The figure shows three views and two pictorial views of one solid part (mm, origin at its lowest corner). Answer the questions. A direction names the side the tool comes from. Coordinates: 2 decimals unless noted, no trailing zeros. Order: outer loops, then holes, each group sorted by start corner. A loop starts at its lowest first (then second) coordinate and runs counter-clockwise, first axis right, second up. Notation, with made-up numbers: (39.25, 1.5) - (52.25, 1.5) arc R21 ccw to (52.25, 7.5) - close; hole circle Ø6 at (-32, 17). An arc over 180 degrees is marked (long way). Answer as a JSON object with one key per item and string values. Group by question number.
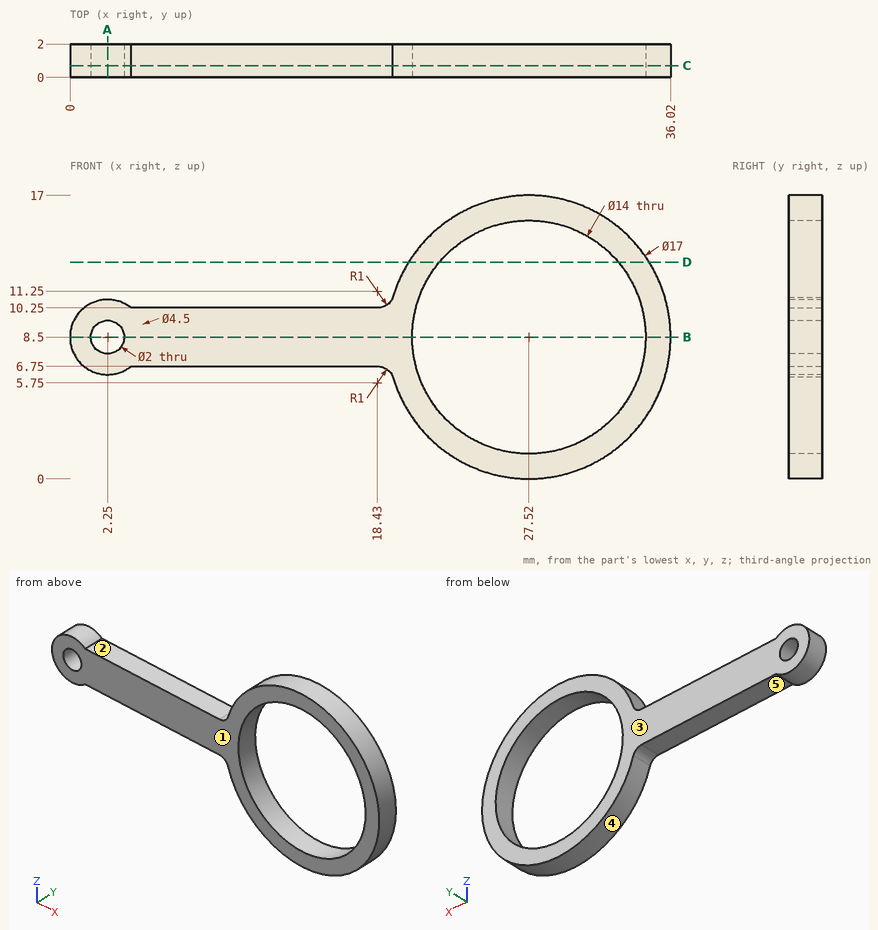
1. A cutting plane is placed at D-D on z = 13. Write down the section's boundary in (x, y), and give its area (3 significant figures).
2. Given pin 1 (1 mm diameter, centred on x = 21.5, y = 1.5, fed in from -Z); pin 2 (1 mm diameter, centred on x = 8.5, y = 1.5, fed in from +Z), each flat-ended and moving along its own axis, determine where each tip first touches the part or whether it passes through.
3. For a pull along X with two mould halves and no side action, classify the marked faces 3, 4 and 5 as pulls with the +X half, pulls with the -X half, needs draft (parallel to the pull), parting line crosses it, or undercut.
4. A cutting plane is placed at B-B on z = 8.5. Write down the section's boundary in (x, y), and give its area (3 significant figures).
5. Straight lines are drawn through the part: L1, parallel to X at y = 0.65, z = 8.5; L2, parallel to X at y = 1.6, z = 10.5; L3, parallel to Z at x = 34, y = 1.25. For each, find the intervals that lie inside material, in ascending order.
6. A cutting plane is placed at A-A on x = 2.25. Write down the section's boundary in (y, z).
7. A cutting plane is placed at C-C on y = 0.7. Write down the section's boundary in (x, z).
8. For the marked faces 1 and 2, determine the directions among +Z, -Z, +X, -X, +Y, -Y from which every point of the face is accessible in a straight line to the end or side of a thin tool.
Derived:
{
 "1": {"outline": "(20.31, 0) - (22.16, 0) - (22.16, 2) - (20.31, 2) - close; (32.88, 0) - (34.73, 0) - (34.73, 2) - (32.88, 2) - close", "area": "7.40 mm2"},
 "2": {"pin 1": "stops at z = 2.04", "pin 2": "stops at z = 10.25"},
 "3": {"face 3": "needs draft", "face 4": "parting line crosses it", "face 5": "undercut"},
 "4": {"outline": "(0, 0) - (1.25, 0) - (1.25, 2) - (0, 2) - close; (3.25, 0) - (20.52, 0) - (20.52, 2) - (3.25, 2) - close; (34.52, 0) - (36.02, 0) - (36.02, 2) - (34.52, 2) - close", "area": "40.0 mm2"},
 "5": {"L1": "x = 0 to 1.25, 3.25 to 20.52, 34.52 to 36.02", "L2": "x = 1.22 to 3.28, 19.09 to 20.81, 34.23 to 35.78", "L3": "z = 3 to 5.85, 11.15 to 14"},
 "6": {"outline": "(0, 6.25) - (2, 6.25) - (2, 7.5) - (0, 7.5) - close; (0, 9.5) - (2, 9.5) - (2, 10.75) - (0, 10.75) - close"},
 "7": {"outline": "(3.66, 6.75) - (18.43, 6.75) arc R1 cw to (19.36, 6.11) arc R8.5 ccw (long way) to (19.36, 10.89) arc R1 cw to (18.43, 10.25) - (3.66, 10.25) arc R2.25 ccw (long way) to start; hole circle Ø2 at (2.25, 8.5); hole circle Ø14 at (27.52, 8.5)"},
 "8": {"face 1": "+Z, -Z, +X, -X, -Y", "face 2": "+Z, +Y, -Y"}
}
